Source: CAD feature listing. Evaluate the final solid. Frame: model axes, mm. Give positions to 0.01 mm unless a question says otherwise; leave off trailing zeros. Write each loop counter-clockwise with the first axis right and the second up, starting at its lowest first coordinate (ties: lowest second). Pieces come first, ordered by that corner, then holes. Notation, with made-up numbers: (-10, 67.25) - (-2, 67.25) arc R24 ccw to (-2, 92.25) - close; hole circle Ø1 at (21, 64). An arc over 180 degrees is marked (long way). One line per question, with ' | ' between items. Start each with the question number.
(1) Pin query (flat end, axial travel): pin 1 (1 mm diameter, centred on y = -40, z = 0.5, fed in from +X); pin 2 (0.6 mm diameter, centred on x = 36.5, z = 1, fed in from +Y); pin 3 (1 mm diameter, centred on y = -39.5, z = 1.5, fed in from -X). Return the tip coordinate at first contact, or that it passes through.
(2) Ray query, line 1 (X direction, y = -45, z = 1.6); line 2 (Y direction, x = 1, z = 1.8); line 3 (X direction, y = -61, z = 0.55). Return the intervals inside material, ascending. Write a range as [from, to].
(3) Section A-A, the plane x = 10.5. Return loops of the section in (y, z), plus the area to 3 significant figures.
```python
from build123d import *

# Parameters (mm, degrees)
RESSALTO_EXTRUS_O1_DEPTH = 2


with BuildPart() as part:
    # Model → Ressalto-extrusão1 (new body)
    with BuildSketch(Plane.XY):
        with BuildLine():
            Line((-58.8502, -40.6768), (-58.8502, -45.1121))
            add(Edge.make_bspline(
                [(-58.8502, -45.1121), (-9.0376, -48.8189), (-12.8956, -79.3194), (-58.8502, -80.0274)],
                knots=[0.047619048, 0.047619048, 0.047619048, 0.047619048, 0.095238095, 0.095238095, 0.095238095, 0.095238095], degree=3))
            Line((-58.8502, -80.0274), (-58.8502, -85.3435))
            Line((-58.8502, -85.3435), (54.4831, -85.3435))
            Line((54.4831, -85.3435), (54.4831, -80.0274))
            add(Edge.make_bspline(
                [(54.4831, -80.0274), (8.5266, -79.3193), (4.6696, -48.8189), (54.4831, -45.1121)],
                knots=[0.238095238, 0.238095238, 0.238095238, 0.238095238, 0.285714286, 0.285714286, 0.285714286, 0.285714286], degree=3))
            Line((54.4831, -45.1121), (54.4831, -40.6768))
            Line((54.4831, -40.6768), (26.1498, -40.6768))
            Line((26.1498, -40.6768), (26.1498, -38.6717))
            Line((26.1498, -38.6717), (19.4831, -38.6717))
            Line((19.4831, -38.6717), (19.4831, -40.6768))
            Line((19.4831, -40.6768), (-1.1835, -40.6768))
            Line((-1.1835, -40.6768), (-1.1835, -61.4949))
            Line((-1.1835, -61.4949), (-3.1835, -61.4949))
            Line((-3.1835, -61.4949), (-3.1835, -40.6768))
            Line((-3.1835, -40.6768), (-23.8502, -40.6768))
            Line((-23.8502, -40.6768), (-23.8502, -38.6717))
            Line((-23.8502, -38.6717), (-30.5169, -38.6717))
            Line((-30.5169, -38.6717), (-30.5169, -40.6768))
            Line((-30.5169, -40.6768), (-58.8502, -40.6768))
        make_face()
    extrude(amount=RESSALTO_EXTRUS_O1_DEPTH)


solid = part.part
```
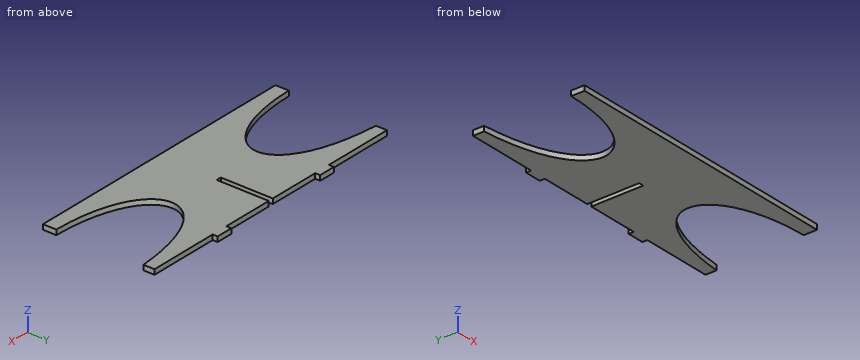
Check sheet entries:
1) pin 1: x = 26.15 | pin 2: y = -40.68 | pin 3: x = -30.52
2) line 1: [-58.85, -3.18], [-1.18, 54.48] | line 2: [-85.34, -40.68] | line 3: [-23.21, -3.18], [-1.18, 18.84]
3) outline: (-85.34, 0) - (-40.68, 0) - (-40.68, 2) - (-85.34, 2) - close | area: 89.3 mm²
